Geometry: final body of the model. Coordinates: model frame, mm. Coordinates: 2 decimals unless noted, no trailing zeros. Write each loop counter-clockwise with the first axis right and the second up, starting at its lowest first coordinate (ties: lowest second). Pieces come first, ordered by that corner, then holes. Notation, with made-up numbers: (52, -1.75) - (97, -1.75) arc R12 ccw to (97, 16.25) - close; hole circle Ø9 at (54, -11.75). An arc over 180 degrees is marked (long way). Answer as a JSON object with one key per item and string values. Group by question number.
Item 1: First-contact query: pin 1 Ø1 at (x, y) = (-13.5, 149) entering from -Z; pin 2 Ø1.5 at (x, z) = (143, 1.5) entering from +Y; pin 3 Ø2 at (x, z) = (61.5, 2) entering from -Y. Flat tips, straight axial feed; report the tip coordinate or a pass-through.
Item 2: Section C-C on y = 117. Return loops of the section in (x, z), and give its area (3 significant figures).
Item 3: Section D-D on x = -102.5. Return loops of the section in (y, z).
Item 4: Line query: line 1 along Y through (x, z) = (17, 3.25); line 2 along Y through (x, z) = (56.5, 0.4); line 3 along Y through (x, z) = (-137.5, 0.3). Output: solid intervals per line, ascending. Write a range as from..to.
Item 5: Section A-A on x = 24. Return loops of the section in (y, z).
Item 6: Section B-B on z = 0.8. State how many separate pieces and enclosed holes the cut face has, and give its area (3 significant figures).
```python
from build123d import *

# Parameters (mm, degrees)
BOSS_EXTRUDE1_DEPTH = 5


with BuildPart() as part:
    # Sketch1 → Boss-Extrude1 (new body)
    with BuildSketch(Plane.XY):
        with BuildLine():
            Line((-83.530674823, -170.653527252), (-74.806628793, -98.304799508))
            ThreePointArc((-74.806628793, -98.304799508), (-5.273873885, -43.7365304), (49.294395236, -113.269285297))
            Line((49.294395236, -113.269285297), (40.570349206, -185.618013041))
            ThreePointArc((40.570349206, -185.618013041), (156.087114581, 108.336571211), (-159.704253129, 102.929837912))
            Line((-159.704253129, 102.929837912), (-150.380705265, 99.896734946))
            Line((-150.380705265, 99.896734946), (-189.050478899, -18.971463523))
            ThreePointArc((-189.050478899, -18.971463523), (-155.971098141, -108.503532406), (-83.530674823, -170.653527252))
        make_face()
        Polygon((-74.257311019, -43.998315425), (-68.970068444, -58.035589589), (-139.156439262, -84.471802466), (-160.305409564, -28.322705811), (-90.119038745, -1.886492934), (-84.83179617, -15.923767097), (-28.682699515, 5.225203205), (-18.108214364, -22.849345123), align=None, mode=Mode.SUBTRACT)
        Polygon((-0.975003372, 86.307875472), (-15.775260686, 88.747626167), (-3.576507208, 162.748912734), (55.624522046, 152.989909952), (43.425768568, 78.988623385), (28.625511255, 81.428374081), (18.866508473, 22.227344827), (-10.734006154, 27.106846218), align=None, mode=Mode.SUBTRACT)
        Polygon((75.232314391, -42.309560047), (84.745329129, -30.712036579), (142.73294647, -78.277110268), (104.680887518, -124.667204141), (46.693270177, -77.102130451), (56.206284915, -65.504606983), (9.816191042, -27.452548031), (28.842220518, -4.257501095), align=None, mode=Mode.SUBTRACT)
    extrude(amount=BOSS_EXTRUDE1_DEPTH)


solid = part.part
```
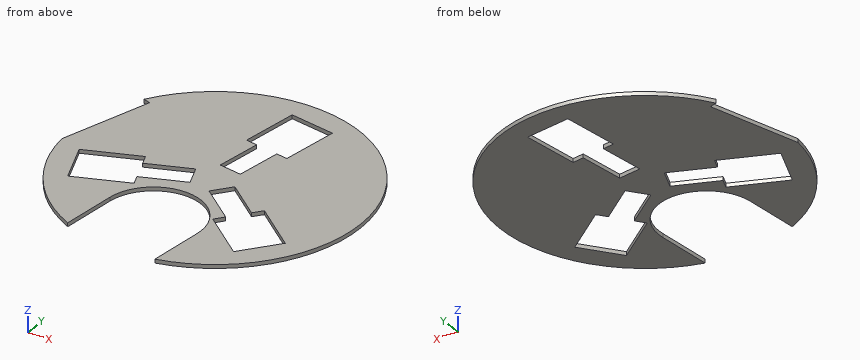
Checks:
{
 "1": {"pin 1": "z = 0", "pin 2": "y = 125.96", "pin 3": "y = -180.11"},
 "2": {"outline": "(-149.7, 0) - (-11.12, 0) - (-11.12, 5) - (-149.7, 5) - close; (49.69, 0) - (149.7, 0) - (149.7, 5) - (49.69, 5) - close", "area": "1,190 mm^2"},
 "3": {"outline": "(-159.98, 0) - (-70.66, 0) - (-70.66, 5) - (-159.98, 5) - close; (-6.55, 0) - (159.98, 0) - (159.98, 5) - (-6.55, 5) - close"},
 "4": {"line 1": "-50.83..-33.35, -18.69..22.54, 159.36..189.24", "line 2": "-181.4..-85.15, -26.94..181.4", "line 3": "-131.12..-83.85, -19.73..131.12"},
 "5": {"outline": "(-55.24, 0) - (-39.09, 0) - (-39.09, 5) - (-55.24, 5) - close; (-10.16, 0) - (53.37, 0) - (53.37, 5) - (-10.16, 5) - close; (158.2, 0) - (188.48, 0) - (188.48, 5) - (158.2, 5) - close"},
 "6": {"separate pieces": "1", "enclosed holes": "3", "area": "76,900 mm^2"}
}
